Drawing for the job (mm, zero at the part's lowest x, y, z). Coordinates: 2 decimals unless noted, no trailing zeros. Order: outer loops, then holes, each group sorted by start corner. A loop starts at its lowest first (then second) coordinate and runs counter-clockwise, first axis right, second up.
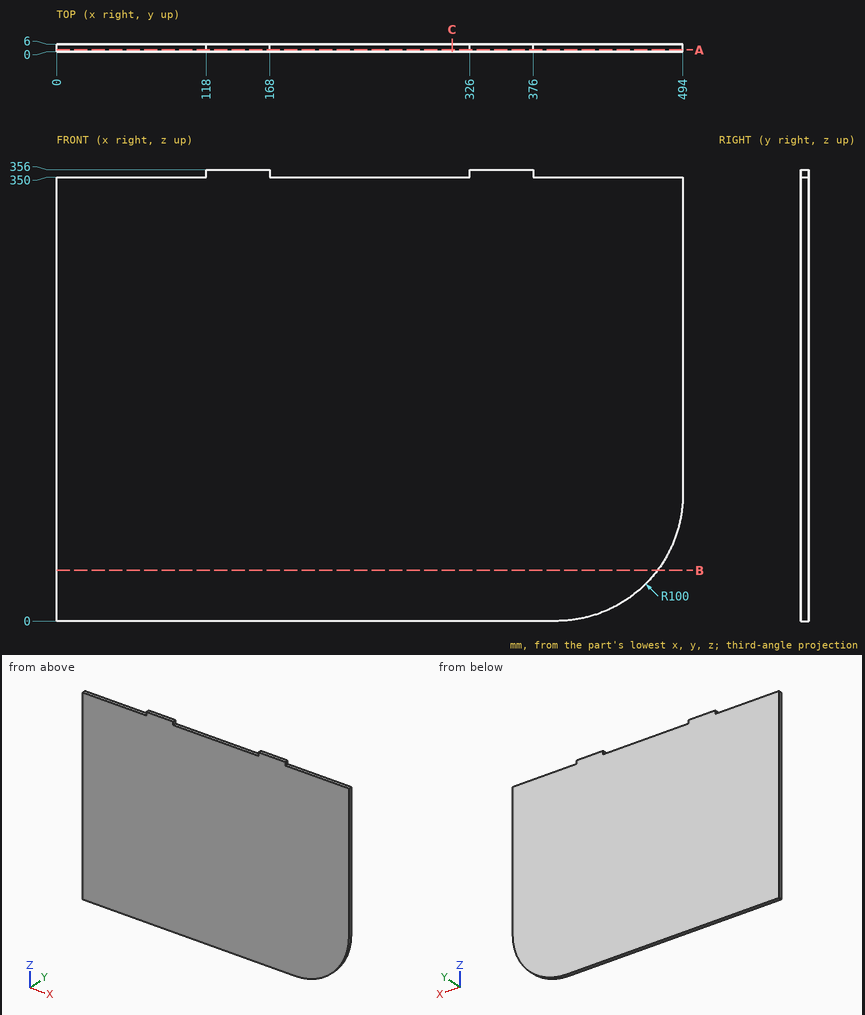
1) Slice it at B-B (z = 40). List the corners of the cut face in (x, y), plus the area to 3 significant figures.
2) Drill centre lines: probe 1 along Z at (x, y) = (112, 0.8); probe 2 along Z at (x, y) = (414, 4.85). Where is each one in solid material? Low to high.
3) Pin check, flat tips, straight feed: P1, Ø2, axis at x = 195, y = 0.5, coming from the -Z side; P2, Ø1.8, axis at y = 2, z = 353, coming from the -X side. Stop position of each tip, or through.
4) Slice it at A-A (y = 1.35). List the corners of the cut face in (x, z), plus the area to 3 significant figures.
5) Slice it at C-C (x = 312). List the corners of the cut face in (y, z), plus the area to 3 significant figures.
Worked out:
1. outline: (0, 0) - (474, 0) - (474, 6) - (0, 6) - close
1. area: 2,840 mm2
2. probe 1: z = 0 to 350
2. probe 2: z = 2.02 to 350
3. P1: stops at z = 0
3. P2: stops at x = 118
4. outline: (0, 0) - (394, 0) arc R100 ccw to (494, 100) - (494, 350) - (376, 350) - (376, 356) - (326, 356) - (326, 350) - (168, 350) - (168, 356) - (118, 356) - (118, 350) - (0, 350) - close
4. area: 171,000 mm2
5. outline: (0, 0) - (6, 0) - (6, 350) - (0, 350) - close
5. area: 2,100 mm2
